Geometry check sheet. Reference: the model listing, model coordinates, mm. Give positions to 0.01 mm unless a question says otherwise; leave off trailing zeros. Write each loop counter-clockwise with the first axis right and the second up, starting at its lowest first coordinate (ties: lowest second). Pieces come first, ordered by that corner, then holes. Notation, with made-up numbers: (86.5, 1) - (102.5, 1) arc R35 ccw to (102.5, 33) - close; hole circle Ø9 at (25.25, 17). An arc over 180 degrees is marked (long way). Write item = value, one per line. Start each with the question number.
(1) Thickness scan on L1, parallel to X at y = 20, z = 0.45; L2, parallel to Y at x = 1, z = 0.25; L3, parallel to X at y = -24.5, z = 0.1. Record the ranges inside material, lowest first.
(2) Depth check by flat-ended pin: pin 1 Ø6 at (x, y) = (-7.5, 4) entering from -Z. Enter the tip coordinate at first touch or a pass-through.
(3) Section check C-C, the plane z = 0.4. Enter the section's corners in (x, y), plus the area to 3 significant figures.
(4) Section check A-A, the plane y = 10. Enter the section's corners in (x, z).
(5) Section check D-D, the plane x = -13. Enter the section's corners in (y, z).
(6) Section check B-B, the plane x = 4.5. Enter the section's corners in (y, z), plus the area to 3 significant figures.
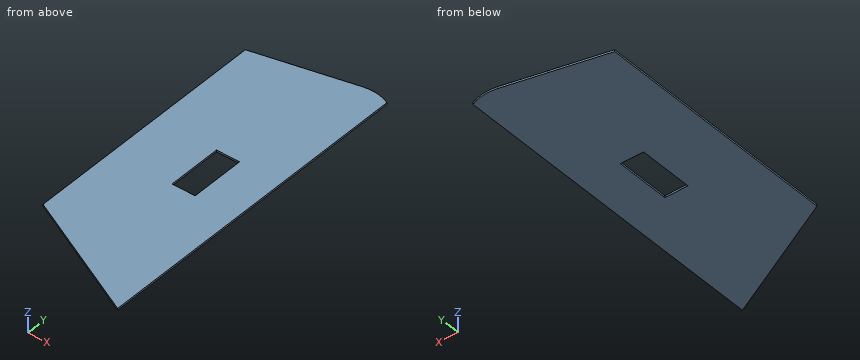
Autodesk Inventor part; units mm, degrees
ref_plane "YZ Plane" through (0, 0, 0) normal (1, 0, 0) x (0, 1, 0)
ref_plane "XZ Plane" through (0, 0, 0) normal (0, 1, 0) x (-1, 0, 0)
ref_plane "XY Plane" through (0, 0, 0) normal (0, 0, 1) x (1, 0, 0)
sketch "Sketch1" plane through (0, 0, 0) normal (0, 0, 1) x (1, 0, 0)
  line L0 (7.5, 3.8038) -> (3.6225, 3.8038)
  arc A0 (1.9153, 4.762) -> (3.6225, 3.8038) centre (3.6225, 5.8038) ccw
  line L1 (1.9153, 4.762) -> (-2.2072, 11.517)
  arc A1 (-2.5, 12.5588) -> (-2.2072, 11.517) centre (-0.5, 12.5588) ccw
  line L2 (-2.5, 12.5588) -> (-2.5, 21.8038)
  arc A2 (-0.5, 23.8038) -> (-2.5, 21.8038) centre (-0.5, 21.8038) ccw
  line L3 (-0.5, 23.8038) -> (7.5, 23.8038)
  line L4 (7.5, 23.8038) -> (7.5, 3.8038)
  spline S0 degree 3 poles (-6.0485, -11.2843) (-6.0213, -11.0209) (-5.9428, -10.7653) (-5.6929, -10.2997) (-5.524, -10.094) (-5.1467, -9.7842) (-4.9505, -9.6718) (-4.5292, -9.5173) (-4.3073, -9.4763) (-4.0832, -9.4731) knots 0 0 0 0 0.079442 0.079442 0.158531 0.158531 0.225919 0.225919 0.293184 0.293184 0.293184 0.293184
  line L5 (-6.0485, -11.2843) -> (-6.563, -16.2598)
  line L6 (-6.563, -16.2598) -> (-6.8849, -19.6266)
  arc A3 (-6.8849, -19.6266) -> (-5.7884, -21.6058) centre (-4.894, -19.817) ccw
  line L7 (17.5, -33.2499) -> (-5.7884, -21.6058)
  line L8 (17.5, 31.9794) -> (17.5, -33.2499)
  arc A4 (4.376, 33.2499) -> (17.5, 31.9794) centre (12.5, 48.7499) ccw
  arc A5 (-1.8324, 56.2463) -> (4.376, 33.2499) centre (12.5, 47.7794) ccw
  line L9 (-1.8324, 56.2463) -> (-17.5, 52.7794)
  line L10 (-17.5, 52.7794) -> (-17.5, 3.0185)
  ellipse E0 centre (-15.5, 3.0185) end of major axis (-15.5, 1.0011) minor radius 2 (-17.5, 3.0185) -> (-15.6888, 1.0101) ccw
  line L11 (-15.6888, 1.0101) -> (-3.1949, -0.1848)
  line L12 (-3.1949, -0.1848) -> (-4.0832, -9.4731)
  circle A6 centre (-12, 26.728) radius 1.25
  circle A7 centre (5.3255, 26.728) radius 1.25
  line L13 (-14, 9.2999) -> (-10, 9.2999)
  line L14 (-14, 15.6999) -> (-14, 9.2999)
  line L15 (-10, 15.6999) -> (-14, 15.6999)
  line L16 (-10, 9.2999) -> (-10, 15.6999)
  line L17 (13.7851, 6.0601) -> (9.7851, 6.0601)
  line L18 (13.7851, -0.3399) -> (13.7851, 6.0601)
  line L19 (9.7851, -0.3399) -> (13.7851, -0.3399)
  line L20 (9.7851, 6.0601) -> (9.7851, -0.3399)
  circle A8 centre (7.1425, -8.6154) radius 1.25
  line L21 (17.5, -33.2499) -> (-17.5, -15.7501)
  line L22 (-17.5, -15.7501) -> (-17.5, -17.9862)
  line L23 (-17.5, -17.9862) -> (17.5, -35.486)
  line L24 (17.5, -35.486) -> (17.5, -33.2499)
  line L25 (-1.4649, 56.8397) -> (-18, 53.1809)
  line L26 (-18, 53.1809) -> (-18, -17.9862)
  line L27 (-18, -17.9862) -> (-17.5, -17.9862)
  line L28 (-17.5, -17.9862) -> (-17.5, 52.7794)
  line L29 (-17.5, 52.7794) -> (-1.8324, 56.2463)
  arc A9 (-1.4649, 56.8397) -> (-1.8324, 56.2463) centre (12.5, 47.7794) ccw
  line L30 (19.5, -37.0206) -> (19.5, 31.9794)
  line L31 (19.5, 31.9794) -> (17.5, 31.9794)
  line L32 (17.5, -37.0206) -> (17.5, 31.9794)
  line L33 (19.5, -37.0206) -> (17.5, -37.0206)
  circle A10 centre (12.5, 47.7794) radius 15.02
  line L34 (-1.4649, 56.8397) -> (-11.9805, 54.5129)
  line L35 (-11.9805, 54.5129) -> (26.5324, 63.5095)
  line L36 (17.5, 31.9794) -> (17.5, 20.7849)
  line L37 (17.5, 20.7849) -> (17.5, 78.444)
  circle A11 centre (12.5, 47.7794) radius 12.1257
  line L38 (-17.5, -15.7501) -> (-17.5, 52.7794)
  line L39 (-1.8324, 56.2463) -> (11.2654, 59.1445)
  line L40 (11.2654, 59.1445) -> (26.5324, 62.5227)
  circle A12 centre (12.5, 47.7794) radius 11.3634
  line L41 (5.8925, 7.1892) -> (-0.5, 7.1892)
  line L42 (-0.5, 7.1892) -> (-0.5, 22.231)
  line L43 (-0.5, 22.231) -> (5.8925, 22.231)
  line L44 (5.8925, 22.231) -> (5.8925, 7.1892)
  point P0 (0, 0)
  point P1 (17.5, 57.9837)
  point P2 (10.0449, 58.8745)
extrude "Extrusion1" add sketch "Sketch1" along normal blind 0.5 contours L0 A0 L1 L41 L44 L43 L42 A1 L2 A2 L3 L4 | L5 L6 A3 L21 L28 E0 L11 L12 S0 | S0 L12 L11 E0 L10 L9 A5 A4 L8 L7 A3 L6 L5 | L39 A10 L37 A4 A5 | L39 A11 L37 A10 | L39 A12 L37 A11 | A12 L37 | L14 L15 L16 L13 | L18 L19 L20 L17 picked at (9.8401, 51.5561)
sketch "Sketch2" plane through (0, 0, 0.5) normal (0, 0, 1) x (1, 0, 0)
  line L0 (17.5, -33.2499) -> (17.5, 57.9837)
  arc A0 (17.5, 57.9837) -> (10.0449, 58.8745) centre (12.5, 47.7794) ccw
  line L1 (10.0449, 58.8745) -> (-17.5, 52.7794)
  line L2 (-17.5, 52.7794) -> (-17.5, -15.7501)
  line L3 (-17.5, -15.7501) -> (17.5, -33.2499)
  circle A1 centre (-12, 26.728) radius 1.25
  circle A2 centre (5.3255, 26.728) radius 1.25
  circle A3 centre (7.1425, -8.6154) radius 1.25
  line L4 (-0.5, 7.1892) -> (-0.5, 22.231)
  line L5 (-0.5, 22.231) -> (5.8925, 22.231)
  line L6 (5.8925, 22.231) -> (5.8925, 7.1892)
  line L7 (5.8925, 7.1892) -> (-0.5, 7.1892)
  point P0 (0, 0)
extrude "Extrusion2" add sketch "Sketch2" against normal blind 0.5 contours A1 | A2 | A3
properties part number "pokrywa lewa" material "Aluminum 6061"
Model answer:
q1.L1 = -17.5 to -0.5, 5.89 to 17.5
q1.L2 = -25 to 7.19, 22.23 to 56.87
q1.L3 = 0 to 17.5
q2.pin_1 = 0
q3.outline = (-17.5, -15.75) - (-5.79, -21.61) - (17.5, -33.25) - (17.5, 57.98) arc R11.36 ccw to (10.04, 58.87) - (-1.83, 56.25) - (-17.5, 52.78) - close; hole (-0.5, 7.19) - (5.89, 7.19) - (5.89, 22.23) - (-0.5, 22.23) - close
q3.area = 2,740 mm²
q4.outline = (-17.5, 0) - (-0.5, 0) - (-0.5, 0.5) - (-17.5, 0.5) - close; (5.89, 0) - (17.5, 0) - (17.5, 0.5) - (5.89, 0.5) - close
q5.outline = (-18, 0) - (53.78, 0) - (53.78, 0.5) - (-18, 0.5) - close
q6.outline = (-26.75, 0) - (7.19, 0) - (7.19, 0.5) - (-26.75, 0.5) - close; (22.23, 0) - (57.65, 0) - (57.65, 0.5) - (22.23, 0.5) - close
q6.area = 34.7 mm²
